from build123d import *

# Parameters (mm, degrees)
SKETCH1_W           = 12.7
SKETCH1_H           = 50.8
BOSS_EXTRUDE1_DEPTH = 12.7
CUT_EXTRUDE1_DEPTH  = 32.108519733
FILLET1_R           = 1.27
SKETCH3_W           = 12.7
SKETCH3_H           = 50.8
SKETCH3_R           = 3.675
BOSS_EXTRUDE2_DEPTH = 6.35


with BuildPart() as part:
    # Sketch1 → Boss-Extrude1 (new body)
    with BuildSketch(Plane.XY):
        Rectangle(SKETCH1_W, SKETCH1_H)
    extrude(amount=BOSS_EXTRUDE1_DEPTH)

    # Sketch2 → Cut-Extrude1 (cut, through all)
    with BuildSketch(Plane(origin=(6.35, 0, 0), x_dir=(0, 0, -1), z_dir=(1, 0, 0))):
        with BuildLine():
            Line((-2.875000092, 19.05), (-2.875000092, -19.05))
            ThreePointArc((-2.875000092, -19.05), (-6.35, -22.524999908), (-9.824999908, -19.05))
            Line((-9.824999908, -19.05), (-9.824999908, 14.904999908))
            Line((-9.824999908, 14.904999908), (-12.7, 14.904999908))
            Line((-12.7, 14.904999908), (-12.7, 22.524999908))
            Line((-12.7, 22.524999908), (-9.824999908, 22.524999908))
            Line((-9.824999908, 22.524999908), (-6.35, 22.524999908))
            ThreePointArc((-6.35, 22.524999908), (-3.892804, 21.507196), (-2.875000092, 19.05))
        make_face()
    extrude(amount=-CUT_EXTRUDE1_DEPTH, mode=Mode.SUBTRACT)

    # Fillet1
    fillet1_edges = [part.edges().sort_by_distance(p)[0] for p in [
        (0, 14.904999908, 9.824999908),
        (0, 14.904999908, 12.7),
        (0, 22.524999908, 12.7),
    ]]
    fillet(fillet1_edges, radius=FILLET1_R)

    # Sketch3 → Boss-Extrude2 (add)
    with BuildSketch(Plane.XZ.offset(25.4)):
        with Locations((0, 6.35)):
            Rectangle(SKETCH3_W, SKETCH3_H)
        with Locations(Location((0, -6.35, 0), (0, 0, 270))):
            Circle(SKETCH3_R, mode=Mode.SUBTRACT)
        with Locations(Location((0, 19.05, 0), (0, 0, 270))):
            Circle(SKETCH3_R, mode=Mode.SUBTRACT)
    extrude(amount=BOSS_EXTRUDE2_DEPTH)


solid = part.part
Geometry check sheet. Reference: the model listing, model coordinates, mm. A direction names the side the tool comes from. Round coordinates to 2 decimals unless told otherwise and drop trailing zeros. Loops run counter-clockwise (first coordinate to the right, second up) from the corner with the lowest first, then second, coordinate; pieces in that order, holes last.
Item 1: Cross-section at B-B on x = 1. Record the boundary of the cut face in (y, z) (3 decimals).
Item 2: Cross-section at C-C on y = 1. Record the boundary of the cut face in (x, z) (3 decimals).
Item 3: Gauge pin test, flat ends, axial feed: pin 1 (0.5 mm diameter, centred on x = -0.5, y = 24.5, fed in from +Z); pin 2 (6.5 mm diameter, centred on x = -1.5, z = 25, fed in from +Y); pin 3 (6 mm diameter, centred on x = -1, y = -19, fed in from -Z). Record the tip position at first contact, or that the pin passes through.
Item 4: Thickness scan on line 1 (X direction, y = -27.5, z = 19.05) (3 decimals); line 2 (Z direction, x = 5.5, y = -1) (3 decimals); line 3 (Z direction, x = 1.5, y = -22). Record the ranges inside material, lowest first.
Item 5: Mould release check, pull along Y, two halves, no side actions. Record for faces 1 (the flat face through (0, -25.4, -12)), 2 (the flat face through (0, 25, 12.7)), 3 (the cylindrical face through (0.089, -22.524, 6.274)): pulls with the +Y half, pulls with the -Y half, needs draft (parallel to the pull), parting line crosses it, or undercut.
Item 6: Access from +Z, -Z, +X, -X, +Y, -Y to the whole of each face (thin tool, end or side, straight path). Record for faces 4 (the flat face through (0, -6, 12.7)), 5 (the flat face through (0, 0, 0)), 6 (the cylindrical face through (-0.089, 14.523, 10.187)), 7 (the flat face through (0, 22.525, 9)).
Item 7: Cross-section at D-D on x = 4.75. Record the boundary of the cut face in (y, z) (3 decimals).
Item 8: Cross-section at A-A on z = 19.05. Record the boundary of the cut face in (x, y) (3 decimals), then the cut area to 3 significant figures.
Answer sheet:
1. outline: (-31.75, -19.05) - (-25.4, -19.05) - (-25.4, -9.886) - (-31.75, -9.886) - close; (-31.75, -2.814) - (-25.4, -2.814) - (-25.4, 0) - (25.4, 0) - (25.4, 12.7) - (23.795, 12.7) arc R1.27 ccw to (22.525, 11.43) - (22.525, 6.35) arc R3.475 cw to (19.05, 2.875) - (-19.05, 2.875) arc R3.475 cw to (-19.05, 9.825) - (13.635, 9.825) arc R1.27 ccw to (14.905, 11.095) - (14.905, 11.43) arc R1.27 ccw to (13.635, 12.7) - (-25.4, 12.7) - (-25.4, 15.514) - (-31.75, 15.514) - close; (-31.75, 22.586) - (-25.4, 22.586) - (-25.4, 31.75) - (-31.75, 31.75) - close
2. outline: (-6.35, 0) - (6.35, 0) - (6.35, 2.875) - (-6.35, 2.875) - close; (-6.35, 9.825) - (6.35, 9.825) - (6.35, 12.7) - (-6.35, 12.7) - close
3. pin 1: stops at z = 12.7
3. pin 2: stops at y = -25.4
3. pin 3: stops at z = 0
4. line 1: x = -6.35 to -3.675, 3.675 to 6.35
4. line 2: z = 0 to 2.875, 9.825 to 12.7
4. line 3: z = 0 to 4.51, 8.19 to 12.7
5. face 1: pulls with the +Y half
5. face 2: needs draft
5. face 3: undercut
6. face 4: +Z, +X, -X, +Y
6. face 5: -Z, +X, -X, +Y
6. face 6: +X, -X
6. face 7: +Z, +X, -X
7. outline: (-31.75, -19.05) - (-25.4, -19.05) - (-25.4, 0) - (25.4, 0) - (25.4, 12.7) - (23.795, 12.7) arc R1.27 ccw to (22.525, 11.43) - (22.525, 6.35) arc R3.475 cw to (19.05, 2.875) - (-19.05, 2.875) arc R3.475 cw to (-19.05, 9.825) - (13.635, 9.825) arc R1.27 ccw to (14.905, 11.095) - (14.905, 11.43) arc R1.27 ccw to (13.635, 12.7) - (-25.4, 12.7) - (-25.4, 31.75) - (-31.75, 31.75) - close
8. outline: (-6.35, -31.75) - (-3.675, -31.75) - (-3.675, -25.4) - (-6.35, -25.4) - close; (3.675, -31.75) - (6.35, -31.75) - (6.35, -25.4) - (3.675, -25.4) - close
8. area: 34.0 mm2
